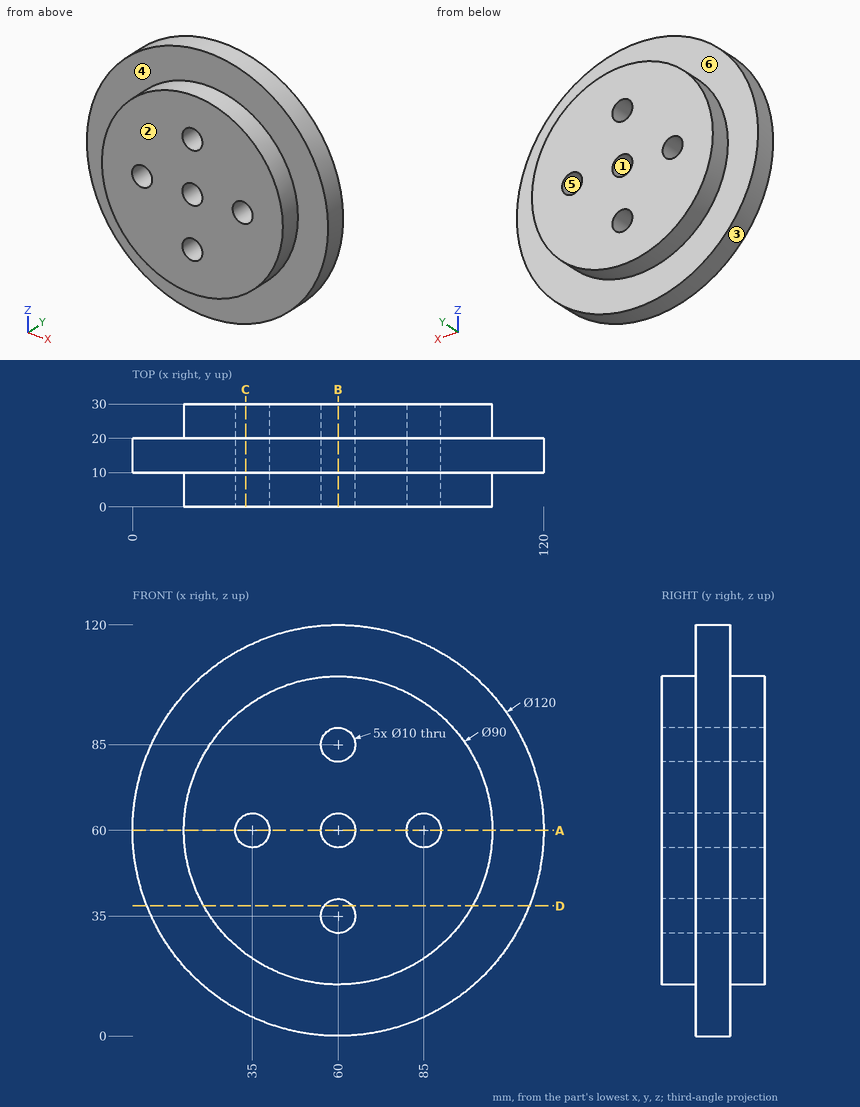
Here's the drawing with two shaded views (mm, measured from the low corner). I have some questions. A direction names the side the tool comes from. Coordinates: 2 decimals unless noted, no trailing zeros. Order: outer loops, then holes, each group sorted by start corner. A loop starts at its lowest first (then second) coordinate and runs counter-clockwise, first axis right, second up. Notation, with made-up numbers: (36, -22.75) -> (80, -22.75) arc R29 cw to (80, 3.25) -> close; hole circle Ø11 at (40, 24). An arc over 180 degrees is marked (long way). Write each question's results on one line, items separated by ' | '.
Item 1: I want a section at B-B, the plane x = 60. Write out the boundary of the cut face in (y, z).
Results are:
outline: (0, 15) -> (10, 15) -> (10, 0) -> (20, 0) -> (20, 15) -> (30, 15) -> (30, 30) -> (0, 30) -> close; (0, 40) -> (30, 40) -> (30, 55) -> (0, 55) -> close; (0, 65) -> (30, 65) -> (30, 80) -> (0, 80) -> close; (0, 90) -> (30, 90) -> (30, 105) -> (20, 105) -> (20, 120) -> (10, 120) -> (10, 105) -> (0, 105) -> close
Item 2: Which directions (+Z, -Z, +X, -X, +Y, -Y) give clear straight access to the entire face, cutting with the end or side of a thin tool? Please do the marked faces 4, 5 and 6.
Results are:
face 4: -Y | face 5: +Y, -Y | face 6: +Y
Item 3: I'm going to push flat-ended pins straight in: pin 1 Ø5 at (x, y) = (105, 16.5) entering from +Z; pin 2 Ø3 at (x, y) = (19.5, 18.5) entering from +Z; pin 3 Ø12 at (x, y) = (16.5, 19.5) entering from -Z. Where does each tip first touch, or does it pass through?
Results are:
pin 1: z = 102.35 | pin 2: z = 105.6 | pin 3: z = 13.16
Item 4: If we mould it in two halves opening along Z, with no side actions, what happens to the marked faces 1, 2 and 3? For each: +Z half, -Z half, draft (parallel to the pull), parting line (faces both ways), or undercut.
Results are:
face 1: undercut | face 2: draft | face 3: parting line
Item 5: If I drill on line 1 along Z through (x, y) = (60, 8.25); line 2 along Y through (x, z) = (71.5, 7); line 3 along Z through (x, y) = (38, 1.75), over which ranges is the centre line in solid material (lowest first)?
Results are:
line 1: 15 to 30, 40 to 55, 65 to 80, 90 to 105 | line 2: 10 to 20 | line 3: 20.74 to 56, 64 to 99.26
Item 6: I want a section at C-C, the plane x = 33. Write out the boundary of the cut face in (y, z).
Results are:
outline: (0, 24) -> (10, 24) -> (10, 6.42) -> (20, 6.42) -> (20, 24) -> (30, 24) -> (30, 55.42) -> (0, 55.42) -> close; (0, 64.58) -> (30, 64.58) -> (30, 96) -> (20, 96) -> (20, 113.58) -> (10, 113.58) -> (10, 96) -> (0, 96) -> close
Item 7: I want a section at A-A, the plane z = 60. Write out the boundary of the cut face in (x, y), then the cut area to 3 significant figures.
Results are:
outline: (0, 10) -> (15, 10) -> (15, 0) -> (30, 0) -> (30, 30) -> (15, 30) -> (15, 20) -> (0, 20) -> close; (40, 0) -> (55, 0) -> (55, 30) -> (40, 30) -> close; (65, 0) -> (80, 0) -> (80, 30) -> (65, 30) -> close; (90, 0) -> (105, 0) -> (105, 10) -> (120, 10) -> (120, 20) -> (105, 20) -> (105, 30) -> (90, 30) -> close | area: 2,100 mm²
Item 8: I want a section at D-D, the plane z = 38. Write out the boundary of the cut face in (x, y), then the cut area to 3 significant figures.
Results are:
outline: (4.18, 10) -> (20.74, 10) -> (20.74, 0) -> (56, 0) -> (56, 30) -> (20.74, 30) -> (20.74, 20) -> (4.18, 20) -> close; (64, 0) -> (99.26, 0) -> (99.26, 10) -> (115.82, 10) -> (115.82, 20) -> (99.26, 20) -> (99.26, 30) -> (64, 30) -> close | area: 2,450 mm²
